```python
from build123d import *

# Parameters (mm, degrees)
SKETCH1_W                  = 100
SKETCH1_H                  = 100
BOSS_EXTRUDE1_DEPTH        = 20
F_12_0_12_DIAMETER_HOLE1_D = 12


with BuildPart() as part:
    # Sketch1 → Boss-Extrude1 (new body)
    with BuildSketch(Plane.XY):
        with Locations((50, 50)):
            Rectangle(SKETCH1_W, SKETCH1_H)
    extrude(amount=-BOSS_EXTRUDE1_DEPTH)

    # Ø12.0 (12) Diameter Hole1 (through all)
    with Locations(Plane.XY):
        with Locations((18.730975853, 16.360822488), (76.507609659, 74.058277502)):
            Hole(F_12_0_12_DIAMETER_HOLE1_D / 2)


solid = part.part
```
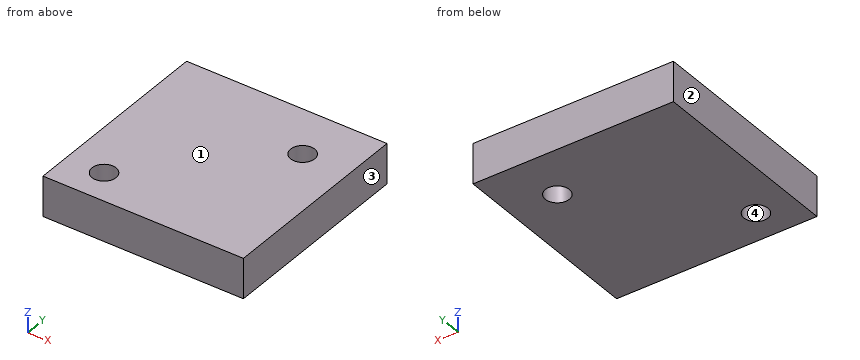
Input: part model. Units: mm. Frame: model coordinates. Face numbers are marked on the shaded views. Coordinates: 2 decimals unless noted, no trailing zeros. Loops run counter-clockwise (first coordinate to the right, second up) from the corner with the lowest first, then second, coordinate; pieces in that order, holes last. Notation, with made-up numbers: M 15,-12.75 L 37,-12.75 A20 ccw 37,8.25 Z; hole C 2.25,65 d1. An arc over 180 degrees is marked long. Answer in a Markdown table with one row per item.
1. Material intervals for line 1 (X direction, y = 16, z = -3); line 2 (Y direction, x = 80.5, z = -6.75); line 3 (Y direction, x = 23, z = -14.75), sorted ascending.
Response:
| item | result |
|---|---|
| line 1 | x = 0 to 12.74, 24.72 to 100 |
| line 2 | y = 0 to 69.58, 78.54 to 100 |
| line 3 | y = 0 to 12.14, 20.58 to 100 |
2. Draft query along X for the marked faces 1, 2, 3 and 4. Return one class per face: pulls with the +X half, pulls with the -X half, needs draft (parallel to the pull), parting line crosses it, or undercut.
Response:
| item | result |
|---|---|
| face 1 | needs draft |
| face 2 | pulls with the -X half |
| face 3 | pulls with the +X half |
| face 4 | undercut |
3. First-contact query: pin 1 (4 mm diameter, centred on x = 66.5, y = 73, fed in from +Z); pin 2 (7 mm diameter, centred on x = 18.73, y = 16.36, fed in from +Z). Flat tips, straight axial feed; report the tip coordinate or a pass-through.
Response:
| item | result |
|---|---|
| pin 1 | stops at z = 0 |
| pin 2 | passes through |
4. Section A-A, the plane x = 76.5. Output: boundary loops of the cut face in (y, z).
Response:
| item | result |
|---|---|
| outline | M 0,-20 L 68.06,-20 L 68.06,0 L 0,0 Z; M 80.06,-20 L 100,-20 L 100,0 L 80.06,0 Z |
5. Section B-B, the plane z = -16.25. Output: boundary loops of the cut face in (x, y), then the cut area to 3 significant figures.
Response:
| item | result |
|---|---|
| outline | M 0,0 L 100,0 L 100,100 L 0,100 Z; hole C 18.73,16.36 d12; hole C 76.51,74.06 d12 |
| area | 9,770 mm2 |
6. Section C-C, the plane x = 18. Output: boundary loops of the cut face in (y, z).
Response:
| item | result |
|---|---|
| outline | M 0,-20 L 10.41,-20 L 10.41,0 L 0,0 Z; M 22.32,-20 L 100,-20 L 100,0 L 22.32,0 Z |
